Read the model definition and answer for the solid it produces. Units are mm, in the model's axes. Round coordinates to 2 decimals unless told otherwise and drop trailing zeros. Loops run counter-clockwise (first coordinate to the right, second up) from the corner with the lowest first, then second, coordinate; pieces in that order, holes last. Notation, with made-up numbers: (34, -31) - (51, -31) arc R20 ccw to (51, -3) - close; hole circle Ø7 at (-10.5, 27). An arc over 180 degrees is marked (long way). Answer as CSV lines item,"result".
```python
from build123d import *

# Parameters (mm, degrees)
CYLINDER005_R     = 1.6
CYLINDER005_DEPTH = 30
PAD002_DEPTH      = 4


with BuildPart() as finger_drill_master:
    # Cylinder005 → Cylinder005 (new body)
    with BuildSketch(Plane.XY.offset(-8)):
        Circle(CYLINDER005_R)
    extrude(amount=CYLINDER005_DEPTH)


with BuildPart() as clone006:
    # Clone006 base: copy of finger-drill-master
    add(finger_drill_master.part)


with BuildPart() as clone006_1:
    # Clone006 placement: moved
    add(clone006.part.moved(Location((40, 0, 0))))


with BuildPart() as fusion012:
    # Clone005 base: copy of finger-drill-master
    add(finger_drill_master.part)

    # Fusion012: union Clone006
    add(clone006_1.part)


with BuildPart() as link_master:
    # Sketch002 → Pad002 (new body)
    with BuildSketch(Plane.XY):
        with BuildLine():
            ThreePointArc((0, 3.7), (-3.7, 0), (0, -3.7))
            Line((0, -3.7), (40, -3.7))
            ThreePointArc((40, -3.7), (43.7, 0), (40, 3.7))
            Line((0, 3.7), (40, 3.7))
        make_face()
    extrude(amount=PAD002_DEPTH)

    # Cut001: cut Fusion012
    add(fusion012.part, mode=Mode.SUBTRACT)


solid = link_master.part
```
1) A cutting plane is placed at A-A, the plane y = 0. Determine the outline of the cut face in (x, z).
Entries:
outline,"(-3.7, 0) - (-1.6, 0) - (-1.6, 4) - (-3.7, 4) - close; (1.6, 0) - (38.4, 0) - (38.4, 4) - (1.6, 4) - close; (41.6, 0) - (43.7, 0) - (43.7, 4) - (41.6, 4) - close"
2) A cutting plane is placed at D-D, the plane y = -2.25. Determine the outline of the cut face in (x, z).
Entries:
outline,"(-2.94, 0) - (42.94, 0) - (42.94, 4) - (-2.94, 4) - close"
3) A cutting plane is placed at C-C, the plane y = 3. Determine the outline of the cut face in (x, z), plus the area to 3 significant figures.
Entries:
outline,"(-2.17, 0) - (42.17, 0) - (42.17, 4) - (-2.17, 4) - close"
area,"177 mm^2"
4) A cutting plane is placed at B-B, the plane z = 3.6. Determine the outline of the cut face in (x, y), plus the area to 3 significant figures.
Entries:
outline,"(0, -3.7) - (40, -3.7) arc R3.7 ccw to (40, 3.7) - (0, 3.7) arc R3.7 ccw to start; hole circle Ø3.2 at (0, 0); hole circle Ø3.2 at (40, 0)"
area,"323 mm^2"
5) Find the intervals of material crossed by line 1 (X direction, y = 0, z = 3.15); line 2 (X direction, y = 0.5, z = 3.8); line 3 (Y direction, x = 0, z = 2.35), in increasing order.
Entries:
line 1,"x = -3.7 to -1.6, 1.6 to 38.4, 41.6 to 43.7"
line 2,"x = -3.67 to -1.52, 1.52 to 38.48, 41.52 to 43.67"
line 3,"y = -3.7 to -1.6, 1.6 to 3.7"
6) The mould has two halves that part along X. Classify faces 1 (the face through (20, 0, 4)), 2 (the face through (-1.27, -0.97, 1.97)), 3 (the face through (43.7, -0.1, 2)): pulls with the +X half, pulls with the -X half, needs draft (parallel to the pull), parting line crosses it, or undercut.
Entries:
face 1,"needs draft"
face 2,"undercut"
face 3,"pulls with the +X half"
